Read the model definition and answer for the solid it produces. Units are mm, in the model's axes. Give positions to 0.01 mm unless a question says otherwise; leave off trailing zeros. Write each loop counter-clockwise with the first axis right and the second up, starting at its lowest first coordinate (ties: lowest second). Pieces come first, ordered by that corner, then holes. Notation, with made-up numbers: M 16.5,15 L 42.5,15 A21 cw 42.5,54 Z; hole C 50.5,43.5 d1. An arc over 180 degrees is marked long. Use a Markdown table: item, result. Add a question column.
Item 1: Consider probe 1 along X at (y, z) = (0.65, -10); probe 2 along Z at (x, y) = (98.1, 1.4); probe 3 along Y at (x, z) = (59.5, -7). Determine where each line is inside the solid, lowest interval first. Write a range as [from, to].
Item 2: A cutting plane is placed at D-D on x = 60. Determine the outline of the cut face in (y, z), then the cut area to 4 significant figures.
Item 3: A cutting plane is placed at B-B on z = -10. Determine the outline of the cut face in (x, y), then the cut area to 3 significant figures.
Item 4: Given P1, Ø10, axis at x = 105.5, z = -24.5, coming from the +Y side; P2, Ø8.5, axis at x = 21.9, z = -10, coming from the -Y side, each flat-ended and moving along its own axis, determine where each tip first touches the part or whether it passes through.
Item 5: A cutting plane is placed at C-C on z = -35. Determine the outline of the cut face in (x, y).
Item 6: A cutting plane is placed at A-A on x = 98.1. Determine the outline of the cut face in (y, z).
Item 7: The mould has two halves that part along Z. Classify faces 1 (the flat face through (120, 1, -20)), 2 (the cylindrical face through (59.2, 15.3, -41.3)), 3 (the cylindrical face through (103.03, 1.52, -7.96)): pulls with the +Z half, pulls with the -Z half, needs draft (parallel to the pull), parting line crosses it, or undercut.
from build123d import *

# Parameters (mm, degrees)
SKETCH1_W           = 120
SKETCH1_H           = 50
BOSS_EXTRUDE1_DEPTH = 3
SKETCH2_R           = 5.334
CUT_EXTRUDE1_DEPTH  = 4
SKETCH3_R           = 6.35
BOSS_EXTRUDE2_DEPTH = 25
FILLET1_R           = 10


with BuildPart() as part:
    # Sketch1 → Boss-Extrude1 (new body)
    with BuildSketch(Plane(origin=(0, 0, 0), x_dir=(1, 0, 0), z_dir=(0, 1, 0))):
        with Locations((60, 25)):
            Rectangle(SKETCH1_W, SKETCH1_H)
    extrude(amount=BOSS_EXTRUDE1_DEPTH)

    # Sketch2 → Cut-Extrude1 (cut, through all)
    with BuildSketch(Plane(origin=(0, 3, 0), x_dir=(1, 0, 0), z_dir=(0, 1, 0))):
        with Locations((21.9, 10)):
            Circle(SKETCH2_R)
        with Locations((98.1, 10)):
            Circle(SKETCH2_R)
    extrude(amount=-CUT_EXTRUDE1_DEPTH, mode=Mode.SUBTRACT)

    # Sketch3 → Boss-Extrude2 (add)
    with BuildSketch(Plane(origin=(0, 3, 0), x_dir=(1, 0, 0), z_dir=(0, 1, 0))):
        with Locations((60, 35)):
            Circle(SKETCH3_R)
    extrude(amount=BOSS_EXTRUDE2_DEPTH)

    # Fillet1
    fillet1_edges = [part.edges().sort_by_distance(p)[0] for p in [
        (0, 1.5, -50),
        (120, 1.5, -50),
    ]]
    fillet(fillet1_edges, radius=FILLET1_R)


solid = part.part
Filled in:
| question | item | result |
|---|---|---|
| 1 | probe 1 | [0, 16.57], [27.23, 92.77], [103.43, 120] |
| 1 | probe 2 | [-50, -15.33], [-4.67, 0] |
| 1 | probe 3 | [0, 3] |
| 2 | outline | M 0,-50 L 3,-50 L 3,-41.35 L 28,-41.35 L 28,-28.65 L 3,-28.65 L 3,0 L 0,0 Z |
| 2 | area | 467.5 mm² |
| 3 | outline | M 0,0 L 16.57,0 L 16.57,3 L 0,3 Z; M 27.23,0 L 92.77,0 L 92.77,3 L 27.23,3 Z; M 103.43,0 L 120,0 L 120,3 L 103.43,3 Z |
| 3 | area | 296 mm² |
| 4 | P1 | y = 3 |
| 4 | P2 | through |
| 5 | outline | M 0,0 L 120,0 L 120,3 L 66.35,3 L 66.35,28 L 53.65,28 L 53.65,3 L 0,3 Z |
| 6 | outline | M 0,-50 L 3,-50 L 3,-15.33 L 0,-15.33 Z; M 0,-4.67 L 3,-4.67 L 3,0 L 0,0 Z |
| 7 | face 1 | needs draft |
| 7 | face 2 | parting line crosses it |
| 7 | face 3 | undercut |
